The listing builds one solid part. Answer for the finished solid, in the listing's coordinates (mm). Give positions to 0.01 mm unless a question says otherwise; leave off trailing zeros. Write each loop counter-clockwise with the first axis right and the second up, starting at its lowest first coordinate (ties: lowest second). Pieces come first, ordered by that corner, then holes. Notation, with made-up numbers: (-25, 52.25) -> (-9, 52.25) arc R24 ccw to (-9, 74.25) -> close; hole circle Ø8 at (63.25, 87). An arc over 180 degrees is marked (long way). Put each result on its own line as item: value. Start each with the question number.
1) For a pull along Y with two mould halves and no side action, classify faces 1 (the cylindrical face through (3.905, 5.675, -0.867)), 2 (the flat face through (-2, 9.99, 0)), 3 (the cylindrical face through (3.105, 0.873, 1.615)) as released by +Y, released by -Y, zero draft, split by the parting line, or undercut.
2) A flat-ended cylindrical pin translates along its axis: pin 1 Ø2 at (y, z) = (1.5, -2) entering from -X. Find the tip coordinate at first contact, or state that the pin passes through.
3) Find the intervals of material crossed by line 1 along Y through (x, z) = (-2, -1); line 2 along Y through (x, z) = (3.75, -1); line 3 along Z through (x, y) = (-1, 4.5), in increasing order. Write a range as from..to.
4) A cutting plane is placed at A-A (y = 7). Write down the section's boundary in (x, z).
from build123d import *

# Parameters (mm, degrees)
CUT_EXTRUDE1_START = -0.01
CUT_EXTRUDE1_DEPTH = 0.01


with BuildPart() as part:
    # Sketch1 → Revolve1 (revolve)
    with BuildSketch(Plane.XY, mode=Mode.PRIVATE) as revolve1_sk:
        with BuildLine():
            Line((0, 0), (0, 10))
            Line((0, 10), (4, 10))
            Line((4, 10), (4, 1.47))
            ThreePointArc((4, 1.47), (3.935563492, 1.314436508), (3.78, 1.25))
            Line((3.78, 1.25), (3.72, 1.25))
            ThreePointArc((3.72, 1.25), (3.564436508, 1.185563492), (3.5, 1.03))
            Line((3.5, 1.03), (3.5, 0.72))
            ThreePointArc((3.5, 0.72), (3.564436508, 0.564436508), (3.72, 0.5))
            Line((3.72, 0.5), (3.78, 0.5))
            ThreePointArc((3.78, 0.5), (3.935563492, 0.435563492), (4, 0.28))
            Line((4, 0.28), (4, 0))
            Line((4, 0), (0, 0))
        make_face()
    revolve(revolve1_sk.sketch.rotate(Axis((0, 10, 0), (0, -1, 0)), 90), axis=Axis((0, 10, 0), (0, -1, 0)))

    # Sketch2 → Cut-Extrude1 (cut)
    with BuildSketch(Plane(origin=(0, 10, 0), x_dir=(1, 0, 0), z_dir=(0, 1, 0)).offset(CUT_EXTRUDE1_START)):
        with BuildLine():
            Line((-1.5, 3.708099244), (-1.5, -3.708099244))
            ThreePointArc((-1.5, -3.708099244), (-4, 0), (-1.5, 3.708099244))
        make_face()
    extrude(amount=CUT_EXTRUDE1_DEPTH, mode=Mode.SUBTRACT)


solid = part.part
Reply:
1. face 1: zero draft
1. face 2: released by +Y
1. face 3: undercut
2. pin 1: stops at x = -3.87
3. line 1: y = 0..9.99
3. line 2: y = 0..0.48, 1.27..10
3. line 3: z = -3.87..3.87
4. outline: circle Ø8 at (0, 0)
